from build123d import *

# Parameters (mm, degrees)
SKETCH_1_W      = 40
SKETCH_1_H      = 40
EXTRUDE_1_DEPTH = 20
FILLET_1_R      = 1
SKETCH_2_R      = 6.5
EXTRUDE_2_DEPTH = 1.5
EXTRUDE_2_TAPER = 15
SKETCH_3_R      = 3
EXTRUDE_3_DEPTH = 3.5
SKETCH_4_R      = 6.5
EXTRUDE_4_DEPTH = 1.5
EXTRUDE_4_TAPER = 15
EXTRUDE_START   = 3.5
SKETCH_5_R      = 3
EXTRUDE_5_DEPTH = 3.5


with BuildPart() as part:
    # 草图1 → 凸台-拉伸1 (new body)
    with BuildSketch(Plane.XY):
        Rectangle(SKETCH_1_W, SKETCH_1_H)
    extrude(amount=EXTRUDE_1_DEPTH)

    # 圆角1
    fillet_1_edges = [part.edges().sort_by_distance(p)[0] for p in [
        (-20, 0, 20),
        (0, -20, 20),
        (20, 0, 20),
        (0, -20, 0),
        (-20, 0, 0),
        (0, 20, 0),
        (20, 0, 0),
        (20, -20, 10),
        (-20, -20, 10),
        (-20, 20, 10),
        (20, 20, 10),
        (0, 20, 20),
    ]]
    fillet(fillet_1_edges, radius=FILLET_1_R)

    # 草图2 → 凸台-拉伸2 (add)
    with BuildSketch(Plane(origin=(0, 20, 0), x_dir=(1, 0, 0), z_dir=(0, 1, 0))):
        with Locations((10, -10)):
            Circle(SKETCH_2_R)
    extrude(amount=EXTRUDE_2_DEPTH, taper=EXTRUDE_2_TAPER)

    # 草图3 → 凸台-拉伸3 (add)
    with BuildSketch(Plane(origin=(0, 21.5, 0), x_dir=(1, 0, 0), z_dir=(0, 1, 0))):
        with Locations(Location((10, -10, 0), (0, 0, 270))):
            Circle(SKETCH_3_R)
    extrude(amount=EXTRUDE_3_DEPTH)

    # 草图4 → 凸台-拉伸4 (add)
    with BuildSketch(Plane.XZ.offset(20)):
        with Locations((10, 10)):
            Circle(SKETCH_4_R)
    extrude(amount=EXTRUDE_4_DEPTH, taper=EXTRUDE_4_TAPER)

    # 草图5 → 凸台-拉伸5 (add)
    with BuildSketch(Plane.XZ.offset(21.5).offset(EXTRUDE_START)):
        with Locations(Location((10, 10, 0), (0, 0, 90))):
            Circle(SKETCH_5_R)
    extrude(amount=-EXTRUDE_5_DEPTH)


solid = part.part
The model under review builds one solid part; all positions refer to its coordinate system, in mm. A direction names the side the tool comes from. Give positions to 0.01 mm unless a question says otherwise; leave off trailing zeros. Order: outer loops, then holes, each group sorted by start corner. A loop starts at its lowest first (then second) coordinate and runs counter-clockwise, first axis right, second up. Notation, with made-up numbers: M 45,67.5 L 90,67.5 A23 cw 90,89.5 Z; hole C -4,39.25 d11. An arc over 180 degrees is marked long. Use one line per item in the form item = value. Start each with the question number.
Item 1: We need section C-C on x = 10. Give the boundary of the cut face in (y, z), plus the area to 3 significant figures.
Item 2: We need section B-B on z = 2.5. Give the boundary of the cut face in (x, y), plus the area to 3 significant figures.
Item 3: We need section A-A on x = 2. Give the boundary of the cut face in (y, z), plus the area to 3 significant figures.
Item 4: For faces 1 (the flat face through (20, 0, 10)), 2 (the flat face through (7, -21.5, 9)), 3 (the cylindrical face through (8.85, 23.23, 12.77)), list the 3-axis set-ups (+Z, -Z, +X, -X, +Y, -Y) from which the entire face can be reached by the end or side of a thin tool; tool diameter is ignored.
Item 5: Insertion check: pin 1 Ø8 at (x, z) = (-13.5, 11) entering from -Y. The pin has a flat end and moves straight along its axis. Give the tip position at first contact, or say it passes through.
Item 6: To check wall thickness, follow line 1 along Y through (x, z) = (1, 12.25); line 2 along Y through (x, z) = (10, 4). State the ranges of each line that lie inside material, in increasing order. Write a range as from..to.
Completed:
q1.outline = M -25,7 L -21.5,7 L -21.5,3.9 L -20,3.5 L -20,1 A1 ccw -19,0 L 19,0 A1 ccw 20,1 L 20,3.5 L 21.5,3.9 L 21.5,7 L 25,7 L 25,13 L 21.5,13 L 21.5,16.1 L 20,16.5 L 20,19 A1 ccw 19,20 L -19,20 A1 ccw -20,19 L -20,16.5 L -21.5,16.1 L -21.5,13 L -25,13 Z
q1.area = 879 mm²
q2.outline = M -20,-19 A1 ccw -19,-20 L 19,-20 A1 ccw 20,-19 L 20,19 A1 ccw 19,20 L -19,20 A1 ccw -20,19 Z
q2.area = 1,600 mm²
q3.outline = M -20,1 A1 ccw -19,0 L 19,0 A1 ccw 20,1 L 20,19 A1 ccw 19,20 L -19,20 A1 ccw -20,19 Z
q3.area = 799 mm²
q4.face_1 = +Z, -Z, +X, +Y, -Y
q4.face_2 = -Y
q4.face_3 = +Y
q5.pin_1 = -20
q6.line_1 = -20..20
q6.line_2 = -21.5..21.5
